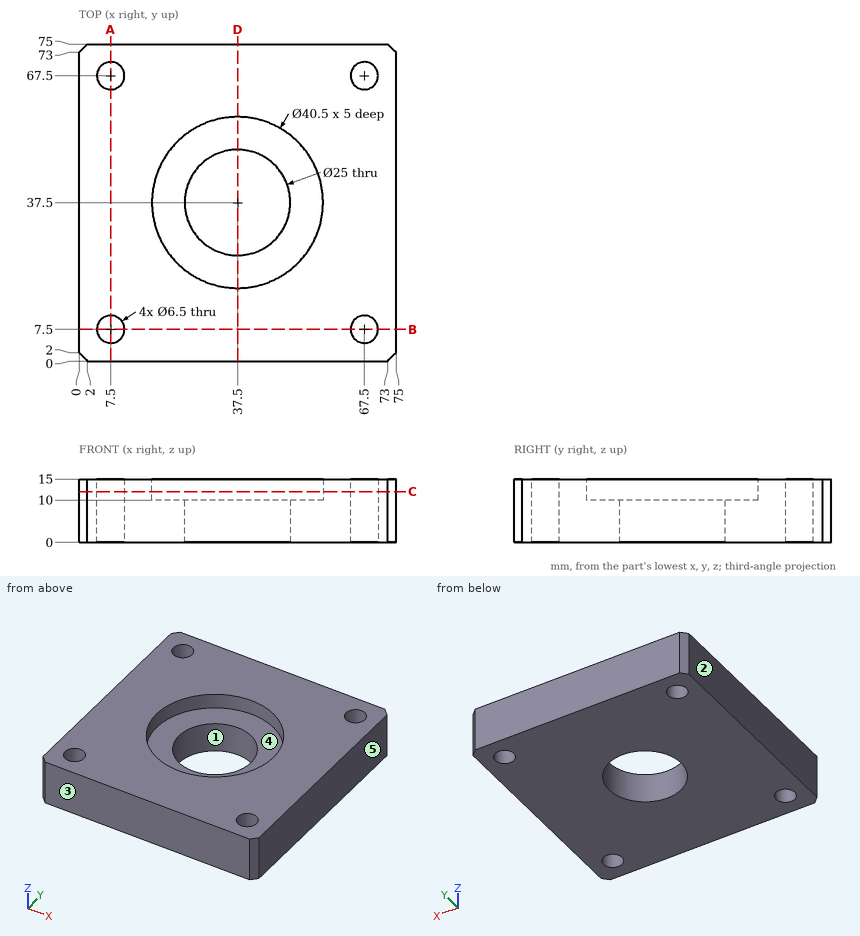
Job drawing, mm, ordinate dimensions from the low corner. One solid piece. A direction names the side the tool comes from. Coordinates: 2 decimals unless noted, no trailing zeros. Order: outer loops, then holes, each group sorted by start corner. A loop starts at its lowest first (then second) coordinate and runs counter-clockwise, first axis right, second up. Notation, with made-up numbers: M 89,-18.5 L 141,-18.5 A22 cw 141,-1.5 Z; hole C 16.25,0 d3. An arc over 180 degrees is marked long. Return JSON: item names as keys, results as strings.
1. Saw through at A-A (x = 7.5). Give the cut face in (y, z).
Ans:
{"outline": "M 0,0 L 4.25,0 L 4.25,15 L 0,15 Z; M 10.75,0 L 64.25,0 L 64.25,15 L 10.75,15 Z; M 70.75,0 L 75,0 L 75,15 L 70.75,15 Z"}
2. Tool access for the marked faces 4 and 5: list every direction of +Z, -Z, +X, -X, +Y, -Y with a clear straight run to the whole face (end or side of a thin tool).
Ans:
{"face 4": "+Z", "face 5": "+Z, -Z, +X, +Y, -Y"}
3. Saw through at D-D (x = 37.5). Give the cut face in (y, z), and give its area (4 significant figures).
Ans:
{"outline": "M 0,0 L 25,0 L 25,10 L 17.25,10 L 17.25,15 L 0,15 Z; M 50,0 L 75,0 L 75,15 L 57.75,15 L 57.75,10 L 50,10 Z", "area": "672.5 mm^2"}
4. Saw through at C-C (z = 12). Give the cut face in (x, y), and give its area (3 significant figures).
Ans:
{"outline": "M 0,2 L 2,0 L 73,0 L 75,2 L 75,73 L 73,75 L 2,75 L 0,73 Z; hole C 7.5,7.5 d6.5; hole C 7.5,67.5 d6.5; hole C 37.5,37.5 d40.5; hole C 67.5,7.5 d6.5; hole C 67.5,67.5 d6.5", "area": "4,200 mm^2"}
5. Drill centre lines: probe 1 along Y at (x, z) = (7.5, 5); probe 2 along Y at (x, z) = (69, 5.5). Where is each one in solid material? Low to high.
Ans:
{"probe 1": "0 to 4.25, 10.75 to 64.25, 70.75 to 75", "probe 2": "0 to 4.62, 10.38 to 64.62, 70.38 to 75"}
6. Flat gauge pin, fed straight in: pin 1 (12 mm diameter, centred on x = 30.5, y = 25.5, fed in from +Z). Where does the tip first touch, or does it go through?
Ans:
{"pin 1": "z = 10"}
7. Pull direction Y, two halves, no side cores. Call the marked faces 1, 2 and 3: +Y half, -Y half, draft (parallel to the pull), parting line (faces both ways), or undercut.
Ans:
{"face 1": "undercut", "face 2": "draft", "face 3": "-Y half"}
